CAD build for the part. Positions are in the model's coordinates, mm. A direction names the side the tool comes from. Coordinates: 2 decimals unless noted, no trailing zeros. Write each loop counter-clockwise with the first axis right and the second up, starting at its lowest first coordinate (ties: lowest second). Pieces come first, ordered by that corner, then holes. Notation, with made-up numbers: (9, 49) - (41, 49) arc R7 ccw to (41, 59) - close; hole circle Ø2 at (-28.5, -24.5). An arc over 180 degrees is marked (long way). Answer in a Markdown table with one row per item. Add a question column.
Q1. Two-plate mould, pull along X, no slides. Class faces 6 (the flat face through (-7, -15, -21.5)), 7 (the flat face through (-6.75, -8, -51)), 8 (the cylindrical face through (-8.67, 14.27, -1.48)): +X half, -X half, draft (parallel to the pull), parting line (faces both ways), or undercut.
Q2. Band-saw the part on C-C (z = -37). List the corners of the cut face in (x, y).
Q3. 3-axis set-ups, long thin cutter, end or side, ignore diameter. For faces 1 (the flat face through (0, -11.5, -51)), 2 (the flat face through (0, -8, -55.5)), 3 (the cylindrical face through (6.83, 14.27, -1.48)), 4 (the flat face through (0, 1, -50)), 5 (the cylindrical face through (-4.01, -18.06, -10.9)): which of +Z, -Z, +X, -X, +Y, -Y reach the whole face in a straight line?
Q4. Band-saw the part on A-A (y = 0). List the corners of the cut face in (x, z).
Q5. Drill centre lines: line 1 along Y through (x, z) = (7, -1); line 2 along Z through (x, y) = (8.5, -14.5); line 3 along Z through (x, y) = (0.5, -12). Where is each one in solid material? Low to high. Write a range as from..to.
Q6. Band-saw the part on B-B (x = 15.5). List the corners of the cut face in (y, z).
Q7. Band-saw the part on D-D (x = -0.5). List the corners of the cut face in (y, z).
Q8. Pin check, flat tips, straight feed: pin 1 (3 mm diameter, centred on x = 7.75, y = 13.42, fed in from -Z); pin 2 (1 mm diameter, centred on x = -2.5, z = 8, fed in from +Y); pin 3 (10 mm diameter, centred on x = -11.5, z = 3.5, fed in from +Y). Stop position of each tip, or through.
```python
from build123d import *

# Parameters (mm, degrees)
EXTRUDE_START          = -21.5
SKETCH_1_R             = 18.5
EXTRUDE_37_21_5_DEPTH  = 21.5
EXTRUDE_START_2        = -44.5
SKETCH_2_R             = 16.4
EXTRUDE_32_8_23_DEPTH  = 23
PCB_START              = -46
SKETCH_3_R             = 16.4
PCB_DEPTH              = 1.5
EXTRUDE_START_3        = -50
SKETCH_4_R             = 6.75
EXTRUDE_504_DEPTH      = 4
XH2_54_START           = -55.5
SKETCH_5_W             = 13.5
SKETCH_5_H             = 7
XH2_54_DEPTH           = 9.5
SKETCH_6_R             = 6
F_7MM_12_DEPTH         = 6
EXTRUDE_START_4        = 6
SKETCH_7_R             = 3
EXTRUDE_6_DEPTH        = 3
EXTRUDE_START_5        = 9
EXTRUDE_D_5_4_12_DEPTH = 12
SKETCH_9_R             = 1.25
F_6XM3_3_DEPTH         = 3


with BuildPart() as part:
    # 草图1 → 减速箱_直径37_长21.5 (new body)
    with BuildSketch(Plane.XY.offset(EXTRUDE_START)):
        Circle(SKETCH_1_R)
    extrude(amount=EXTRUDE_37_21_5_DEPTH)

    # 草图2 → 电机壳_直径32.8_长23 (add)
    with BuildSketch(Plane.XY.offset(EXTRUDE_START_2)):
        Circle(SKETCH_2_R)
    extrude(amount=EXTRUDE_32_8_23_DEPTH)

    # 草图3 → 编码器PCB (add)
    with BuildSketch(Plane.XY.offset(PCB_START)):
        Circle(SKETCH_3_R)
    extrude(amount=PCB_DEPTH)

    # 草图4 → Extrude 504 (add)
    with BuildSketch(Plane.XY.offset(EXTRUDE_START_3)):
        Circle(SKETCH_4_R)
    extrude(amount=EXTRUDE_504_DEPTH)

    # 草图5 → XH2.54连接器_外形简化 (add)
    with BuildSketch(Plane.XY.offset(XH2_54_START)):
        with Locations((0, -8)):
            Rectangle(SKETCH_5_W, SKETCH_5_H)
    extrude(amount=XH2_54_DEPTH)

    # 草图6 → 偏心7mm_轴台直径12 (add)
    with BuildSketch(Plane.XY):
        with Locations((0, 7)):
            Circle(SKETCH_6_R)
    extrude(amount=F_7MM_12_DEPTH)

    # 草图7 → 输出轴直径6 (add)
    with BuildSketch(Plane.XY.offset(EXTRUDE_START_4)):
        with Locations((0, 7)):
            Circle(SKETCH_7_R)
    extrude(amount=EXTRUDE_6_DEPTH)

    # 草图8 → D轴_5.4对边_削平长12 (add)
    with BuildSketch(Plane.XY.offset(EXTRUDE_START_5)):
        with BuildLine():
            Line((2.4, 5.2), (2.4, 8.8))
            ThreePointArc((2.4, 8.8), (-3, 7), (2.4, 5.2))
        make_face()
    extrude(amount=EXTRUDE_D_5_4_12_DEPTH)

    # 草图9 → 6xM3安装底孔_深3_牙型简化 (cut)
    with BuildSketch(Plane.XY):
        with Locations((15.5, 0)):
            Circle(SKETCH_9_R)
        with Locations((7.75, 13.423393759)):
            Circle(SKETCH_9_R)
        with Locations((-7.75, 13.423393759)):
            Circle(SKETCH_9_R)
        with Locations((-15.5, 0)):
            Circle(SKETCH_9_R)
        with Locations((-7.75, -13.423393759)):
            Circle(SKETCH_9_R)
        with Locations((7.75, -13.423393759)):
            Circle(SKETCH_9_R)
    extrude(amount=-F_6XM3_3_DEPTH, mode=Mode.SUBTRACT)


solid = part.part
```
Checked values:
| question | item | result |
|---|---|---|
| 1 | face 6 | draft |
| 1 | face 7 | -X half |
| 1 | face 8 | undercut |
| 2 | outline | circle Ø32.8 at (0, 0) |
| 3 | face 1 | -Z, +X, -X, -Y |
| 3 | face 2 | -Z, +X, -X, +Y, -Y |
| 3 | face 3 | +Z |
| 3 | face 4 | -Z, +X, -X, +Y |
| 3 | face 5 | +Z, -Z |
| 4 | outline | (-18.5, -21.5) - (-16.4, -21.5) - (-16.4, -46) - (-6.75, -46) - (-6.75, -50) - (6.75, -50) - (6.75, -46) - (16.4, -46) - (16.4, -21.5) - (18.5, -21.5) - (18.5, 0) - (16.75, 0) - (16.75, -3) - (14.25, -3) - (14.25, 0) - (-14.25, 0) - (-14.25, -3) - (-16.75, -3) - (-16.75, 0) - (-18.5, 0) - close |
| 5 | line 1 | y = -17.12..-14.42, -12.42..12.42, 14.42..17.12 |
| 5 | line 2 | z = -21.5..0 |
| 5 | line 3 | z = -46..0 |
| 6 | outline | (-10.1, -21.5) - (-5.36, -21.5) - (-5.36, -46) - (5.36, -46) - (5.36, -21.5) - (10.1, -21.5) - (10.1, 0) - (1.25, 0) - (1.25, -3) - (-1.25, -3) - (-1.25, 0) - (-10.1, 0) - close |
| 7 | outline | (-18.49, -21.5) - (-16.39, -21.5) - (-16.39, -46) - (-11.5, -46) - (-11.5, -55.5) - (-4.5, -55.5) - (-4.5, -50) - (6.73, -50) - (6.73, -46) - (16.39, -46) - (16.39, -21.5) - (18.49, -21.5) - (18.49, 0) - (12.98, 0) - (12.98, 6) - (9.96, 6) - (9.96, 21) - (4.04, 21) - (4.04, 6) - (1.02, 6) - (1.02, 0) - (-18.49, 0) - close |
| 8 | pin 1 | stops at z = -46 |
| 8 | pin 2 | stops at y = 9.24 |
| 8 | pin 3 | stops at y = 16.71 |
